from build123d import *

# Parameters (mm, degrees)
ESQUISSE1_R               = 1.5
ESQUISSE1_W               = 23
ESQUISSE1_H               = 12.5
ESQUISSE1_W_2             = 3.2
ESQUISSE1_H_2             = 6
ESQUISSE1_H_3             = 4.2
ESQUISSE1_W_3             = 10
ESQUISSE1_H_4             = 3.2
ESQUISSE1_W_4             = 15
ESQUISSE1_H_5             = 3.3
ESQUISSE1_W_5             = 3
ESQUISSE1_H_6             = 4.3
ESQUISSE1_H_7             = 2.3
T_LE_DE_BASE_PLI_E1_DEPTH = 3


# Sheet-metal steps are written as plain solids
with BuildPart() as part:
    # Esquisse1 → Tôle de base pliée1 (new body)
    with BuildSketch(Plane.XY):
        with BuildLine():
            Line((-822.16567012, 1708.277520055), (-768.16567012, 1708.277520055))
            ThreePointArc((-768.16567012, 1708.277520055), (-766.044349777, 1707.398840398), (-765.16567012, 1705.277520055))
            Line((-765.16567012, 1705.277520055), (-765.16567012, 1667.777520055))
            ThreePointArc((-765.16567012, 1667.777520055), (-766.044349777, 1665.656199711), (-768.16567012, 1664.777520055))
            Line((-768.16567012, 1664.777520055), (-822.16567012, 1664.777520055))
            ThreePointArc((-822.16567012, 1664.777520055), (-824.286990464, 1665.656199711), (-825.16567012, 1667.777520055))
            Line((-825.16567012, 1667.777520055), (-825.16567012, 1705.277520055))
            ThreePointArc((-825.16567012, 1705.277520055), (-824.286990464, 1707.398840398), (-822.16567012, 1708.277520055))
        make_face()
        with Locations((-785.66567012, 1706.077520055)):
            Circle(ESQUISSE1_R, mode=Mode.SUBTRACT)
        with Locations((-785.66567012, 1686.177520055)):
            Circle(ESQUISSE1_R, mode=Mode.SUBTRACT)
        with Locations((-820.91567012, 1675.727520055)):
            Circle(ESQUISSE1_R, mode=Mode.SUBTRACT)
        with Locations((-769.36567012, 1676.127520055)):
            Circle(ESQUISSE1_R, mode=Mode.SUBTRACT)
        with Locations((-785.66567012, 1696.527520055)):
            Rectangle(ESQUISSE1_W, ESQUISSE1_H, mode=Mode.SUBTRACT)
        with Locations((-820.86567012, 1682.277520055)):
            Rectangle(ESQUISSE1_W_2, ESQUISSE1_H_2, mode=Mode.SUBTRACT)
        with Locations((-820.86567012, 1668.477520055)):
            Rectangle(ESQUISSE1_W_2, ESQUISSE1_H_3, mode=Mode.SUBTRACT)
        with Locations((-812.71567012, 1670.877520055)):
            Rectangle(ESQUISSE1_W_3, ESQUISSE1_H_4, mode=Mode.SUBTRACT)
        with Locations((-779.91567012, 1671.027520055)):
            Rectangle(ESQUISSE1_W_4, ESQUISSE1_H_5, mode=Mode.SUBTRACT)
        with Locations((-769.36567012, 1668.627520055)):
            Rectangle(ESQUISSE1_W_5, ESQUISSE1_H_6, mode=Mode.SUBTRACT)
        with Locations((-769.36567012, 1680.727520055)):
            Rectangle(ESQUISSE1_W_5, ESQUISSE1_H_7, mode=Mode.SUBTRACT)
        with Locations((-769.36567012, 1684.427520055)):
            Rectangle(ESQUISSE1_W_5, ESQUISSE1_H_7, mode=Mode.SUBTRACT)
    extrude(amount=-T_LE_DE_BASE_PLI_E1_DEPTH)


solid = part.part
Verification items for the finished model (mm, model axes). A direction names the side the tool comes from. Give positions to 0.01 mm unless a question says otherwise; leave off trailing zeros. Write each loop counter-clockwise with the first axis right and the second up, starting at its lowest first coordinate (ties: lowest second). Pieces come first, ordered by that corner, then holes. Notation, with made-up numbers: (48, 88.25) -> (61, 88.25) arc R9 cw to (61, 105.25) -> close; hole circle Ø11 at (18.5, -38.5). An arc over 180 degrees is marked (long way). Use CSV: the item, a comma, the result in double quotes.
(1) Sectioned sample at C-C (y = 1693). Record the cut outline in (x, z), plus the area to 3 significant figures.
Derived:
outline,"(-825.17, -3) -> (-797.17, -3) -> (-797.17, 0) -> (-825.17, 0) -> close; (-774.17, -3) -> (-765.17, -3) -> (-765.17, 0) -> (-774.17, 0) -> close"
area,"111 mm^2"
(2) Sectioned sample at A-A (y = 1681). Record the cut outline in (x, z).
Derived:
outline,"(-825.17, -3) -> (-822.47, -3) -> (-822.47, 0) -> (-825.17, 0) -> close; (-819.27, -3) -> (-770.87, -3) -> (-770.87, 0) -> (-819.27, 0) -> close; (-767.87, -3) -> (-765.17, -3) -> (-765.17, 0) -> (-767.87, 0) -> close"
(3) Sectioned sample at D-D (x = -778.5). Record the cut outline in (y, z).
Derived:
outline,"(1664.78, -3) -> (1669.38, -3) -> (1669.38, 0) -> (1664.78, 0) -> close; (1672.68, -3) -> (1690.28, -3) -> (1690.28, 0) -> (1672.68, 0) -> close; (1702.78, -3) -> (1708.28, -3) -> (1708.28, 0) -> (1702.78, 0) -> close"
(4) Material ranges on L1, parallel to Y at x = -778, z = -0.4; L2, parallel to X at y = 1671.5, z = -2.35; L3, parallel to X at y = 1669.5, z = -2.35, recorded low to high.
Derived:
L1,"y = 1664.78 to 1669.38, 1672.68 to 1690.28, 1702.78 to 1708.28"
L2,"x = -825.17 to -817.72, -807.72 to -787.42, -772.42 to -765.17"
L3,"x = -825.17 to -822.47, -819.27 to -817.72, -807.72 to -787.42, -772.42 to -770.87, -767.87 to -765.17"
(5) Sectioned sample at B-B (x = -792). Record the cut outline in (y, z).
Derived:
outline,"(1664.78, -3) -> (1690.28, -3) -> (1690.28, 0) -> (1664.78, 0) -> close; (1702.78, -3) -> (1708.28, -3) -> (1708.28, 0) -> (1702.78, 0) -> close"
(6) Release check for a two-part mould opening along X. For faces 1 (the flat face through (-769, 1683.278, -1)), 2 (the flat face through (-795, 1664.778, -1)), 3 (the cylindrical face through (-824.26, 1665.63, -1.48)) record: +X half, -X half, draft (parallel to the pull), parting line (faces both ways), or undercut.
Derived:
face 1,"undercut"
face 2,"draft"
face 3,"-X half"
(7) Set-up check for faces 4 (the cylindrical face through (-824.31, 1707.375, -1.479)), 5 (the flat face through (-770.866, 1681, -1)): record each of +Z, -Z, +X, -X, +Y, -Y from which the full face is reachable in a straight line by a thin tool's end or side.
Derived:
face 4,"+Z, -Z, -X, +Y"
face 5,"+Z, -Z"
